Here's how the part is built. I have some questions about the finished solid (model axes, mm). Face numbers are marked on the shaded views. A direction names the side the tool comes from. Coordinates: 2 decimals unless noted, no trailing zeros. Write each loop counter-clockwise with the first axis right and the second up, starting at its lowest first coordinate (ties: lowest second). Pieces come first, ordered by that corner, then holes. Notation, with made-up numbers: (16, -17) - (65, -17) arc R38 ccw to (65, 21) - close; hole circle Ø8 at (1, 9). An arc over 180 degrees is marked (long way). Answer in a Markdown table with one row per item. Add a question column.
Item 1: Imagine slicing it at C-C (z = 4.5). Please give me the cut outline in (x, y).
Item 2: We'd pull the mould along Y, two halves only. Please class the marked faces 4, 5 and 6: +Y half, -Y half, draft (parallel to the pull), parting line (faces both ways), or undercut.
Item 3: If I drill on probe 1 along Z at (x, y) = (-7, 9.5); probe 2 along Y at (x, z) = (11, -4.75); probe 3 along X at (y, z) = (-11, -1.75), over which ranges is the centre line in solid material (lowest first)? Write a range as from..to.
Item 4: Imagine slicing it at A-A (z = -5). Please give me the cut outline in (x, y), plus the area to 3 significant figures.
Item 5: Imagine slicing it at B-B (y = 0). Please give me the cut outline in (x, z), plus the area to 3 significant figures.
Item 6: Which directions (+Z, -Z, +X, -X, +Y, -Y) give clear straight access to the entire face, cutting with the end or side of a thin tool? Please do the marked faces 1, 2 and 3.
Item 7: I'm going to push flat-ended pins straight in: pin 1 (6 mm diameter, centred on y = -8.5, z = -6, fed in from -X); pin 2 (6 mm diameter, centred on x = -11.5, z = -5, fed in from -Y); pin 3 (1.5 mm diameter, centred on x = 5.5, z = 4.5, fed in from +Y). Where does each tip first touch, or does it pass through?
from build123d import *

# Parameters (mm, degrees)
SKETCH_1_R          = 15
EXTRUDE_1_DEPTH     = 6.5
SKETCH_2_R          = 21
EXTRUDE_2_DEPTH     = 8.5
SKETCH_3_R          = 1.6
CUT_EXTRUDE_1_DEPTH = 26.5
SKETCH_6_W          = 15
SKETCH_6_H          = 50
CUT_EXTRUDE_3_DEPTH = 7.5
FILLET_1_R          = 1
SKETCH_7_R          = 21
SKETCH_7_R_2        = 17
CUT_EXTRUDE_4_DEPTH = 2
FILLET_2_R          = 1


with BuildPart() as part:
    # 草图1 → 凸台-拉伸1 (new body)
    with BuildSketch(Plane.XY):
        with Locations(Location((0, 0, 0), (0, 0, 180))):
            Circle(SKETCH_1_R)
    extrude(amount=EXTRUDE_1_DEPTH)

    # 草图2 → 凸台-拉伸2 (add)
    with BuildSketch(Plane(origin=(0, 0, 0), x_dir=(-1, 0, 0), z_dir=(0, 0, -1))):
        Circle(SKETCH_2_R)
    extrude(amount=EXTRUDE_2_DEPTH)

    # 草图3 → 切除-拉伸1 (cut)
    with BuildSketch(Plane(origin=(0, 0, -8.5), x_dir=(-1, 0, 0), z_dir=(0, 0, -1))):
        with Locations((0, 13.5)):
            Circle(SKETCH_3_R)
        with Locations((11.691342951, -6.75)):
            Circle(SKETCH_3_R)
        with Locations((-11.691342951, -6.75)):
            Circle(SKETCH_3_R)
    extrude(amount=-CUT_EXTRUDE_1_DEPTH, mode=Mode.SUBTRACT)

    # 草图6 → 切除-拉伸3 (cut)
    with BuildSketch(Plane(origin=(0, 0, -8.5), x_dir=(-1, 0, 0), z_dir=(0, 0, -1))):
        Rectangle(SKETCH_6_W, SKETCH_6_H)
    extrude(amount=-CUT_EXTRUDE_3_DEPTH, mode=Mode.SUBTRACT)

    # 圆角1
    # the kernel refuses this fillet: 1 mm, written as the material it takes off along each edge
    with BuildSketch(Plane(origin=(-0.586781578, 14.988518519, 11.997469711), x_dir=(-0.6032076462892466, -0.7975841870662852, 0), z_dir=(0, 0, -1)), Plane(origin=(-12.687047013, -8.002427012, 11.997469711), x_dir=(0.9923319908008487, -0.1236010519098617, 0), z_dir=(0, 0, -1)), Plane(origin=(13.273828591, -6.986091506, 11.997469711), x_dir=(-0.38912434451096145, 0.9211852389768925, 0), z_dir=(0, 0, -1))) as fillet_1_piece_1:
        with BuildLine():
            CenterArc((2.187327708, 0.853683412), FILLET_1_R, 132.251057191, 106.363529617)
            ThreePointArc((1.514947242, 1.593889134), (0.728226426, 0.824743212), (0, 0))
            ThreePointArc((0, 0), (0.833267698, 0.23410654), (1.666535396, 0))
        make_face()
    extrude(amount=11.997469711, mode=Mode.SUBTRACT)
    with BuildSketch(Plane(origin=(0.586781578, 14.988518519, 11.997469711), x_dir=(0.6032076462892473, -0.7975841870662848, 0), z_dir=(0, 0, -1))) as fillet_1_piece_2:
        with BuildLine():
            CenterArc((2.187327708, -0.853683412), FILLET_1_R, 121.385413192, 106.363529617)
            ThreePointArc((1.514947242, -1.593889134), (0.728226426, -0.824743212), (0, 0))
            ThreePointArc((0, 0), (0.833267698, -0.23410654), (1.666535396, 0))
        make_face()
    extrude(amount=11.997469711, mode=Mode.SUBTRACT)
    with BuildSketch(Plane(origin=(-13.273828591, -6.986091506, 11.997469711), x_dir=(-0.3996221607245731, 0.9166799488686461, 0), z_dir=(0, 0, -1)), Plane(origin=(12.687047013, -8.002427012, 11.997469711), x_dir=(-0.594057042497704, -0.8044229175370883, 0), z_dir=(0, 0, -1))) as fillet_1_piece_3:
        with BuildLine():
            CenterArc((2.125688288, 0.997309966), FILLET_1_R, 167.839997769, 106.363529617)
            ThreePointArc((1.148125108, 1.207952385), (0.743749651, 0.442693331), (0, 0))
            ThreePointArc((0, 0), (1.099493942, -0.040350503), (2.198987885, 0))
        make_face()
    extrude(amount=11.997469711, mode=Mode.SUBTRACT)

    # 草图7 → 切除-拉伸4 (cut)
    with BuildSketch(Plane.XY):
        Circle(SKETCH_7_R)
        Circle(SKETCH_7_R_2, mode=Mode.SUBTRACT)
    extrude(amount=-CUT_EXTRUDE_4_DEPTH, mode=Mode.SUBTRACT)

    # 圆角2
    fillet_2_edges = [part.edges().sort_by_distance(p)[0] for p in [
        (-17, 0, -2),
        (14.43086969, -8.986100378, -2),
    ]]
    fillet(fillet_2_edges, radius=FILLET_2_R)


solid = part.part
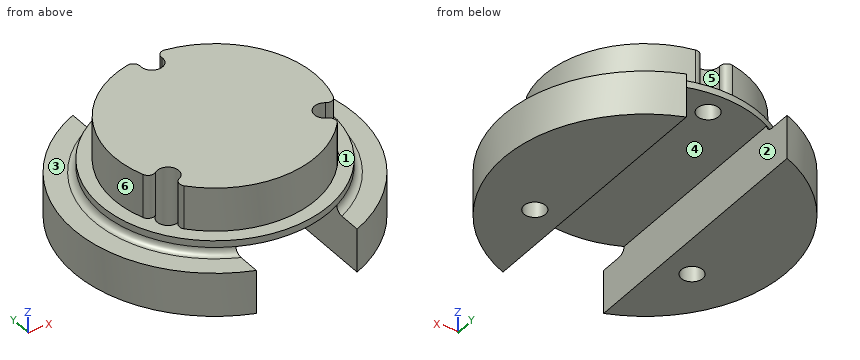
Here are the results:
| question | item | result |
|---|---|---|
| 1 | outline | (-14.15, -4.97) arc R1 ccw to (-12.63, -5.45) arc R1.6 cw (long way) to (-11.03, -8.21) arc R1 ccw to (-11.38, -9.77) arc R15 ccw to (11.38, -9.77) arc R1 ccw to (11.03, -8.21) arc R1.6 cw (long way) to (12.63, -5.45) arc R1 ccw to (14.15, -4.97) arc R15 ccw to (2.77, 14.74) arc R1 ccw to (1.59, 13.66) arc R1.6 cw (long way) to (-1.59, 13.66) arc R1 ccw to (-2.77, 14.74) arc R15 ccw to start |
| 2 | face 4 | draft |
| 2 | face 5 | undercut |
| 2 | face 6 | parting line |
| 3 | probe 1 | z = -1..6.5 |
| 3 | probe 2 | y = -17.89..-8.19, -5.31..17.89 |
| 3 | probe 3 | x = -13.4..-7.5, 7.5..13.4 |
| 4 | outline | (-7.5, -19.62) - (-7.5, 19.62) arc R21 ccw to start; (7.5, -19.62) arc R21 ccw to (7.5, 19.62) - close; hole circle Ø3.2 at (-11.69, -6.75); hole circle Ø3.2 at (11.69, -6.75) |
| 4 | area | 753 mm2 |
| 5 | outline | (-21, -8.5) - (-7.5, -8.5) - (-7.5, -1) - (7.5, -1) - (7.5, -8.5) - (21, -8.5) - (21, -2) - (18, -2) arc R1 cw to (17, -1) - (17, 0) - (15, 0) - (15, 6.5) - (-15, 6.5) - (-15, 0) - (-17, 0) - (-17, -1) arc R1 cw to (-18, -2) - (-21, -2) - close |
| 5 | area | 424 mm2 |
| 6 | face 1 | +Z |
| 6 | face 2 | -Z, +Y, -Y |
| 6 | face 3 | +Z, -X |
| 7 | pin 1 | stops at x = -20.27 |
| 7 | pin 2 | stops at y = -19.2 |
| 7 | pin 3 | stops at y = 14.23 |
